Source: CAD feature listing. Evaluate the final solid. Frame: model axes, mm. Face numbers are marked on the shaded views. A direction names the side the tool comes from. Round coordinates to 2 decimals unless told otherwise and drop trailing zeros. Loops run counter-clockwise (first coordinate to the right, second up) from the corner with the lowest first, then second, coordinate; pieces in that order, holes last.
(1) Section D-D, the plane z = -1. Return the cut outline in (x, y) (3 decimals), plus the area to 3 significant figures.
(2) Set-up query: the marked faces 1, 2 and 3. Return all of +Z, -Z, +X, -X, +Y, -Y with unobstructed straight access to the full face (end or side cutting, diameter ignored); none if empty.
(3) Mould query, pull axis Y, two halves, no side actions, for the marked faces 4, 5, 6 and 7. Classes: pulls with the +Y half, pulls with the -Y half, needs draft (parallel to the pull), parting line crosses it, or undercut.
(4) Section A-A, the plane z = -6. Return the cut outline in (x, y) (3 decimals).
(5) Section C-C, the plane z = -23.83. Return the cut outline in (x, y) (3 decimals), plus the area to 3 significant figures.
(6) Section B-B, the plane x = 0. Return the cut outline in (y, z) (3 decimals), plus the area to 3 significant figures.
(7) First-contact query: pin 1 Ø8 at (x, y) = (-8, 2.5) entering from -Z; pin 2 Ø7.5 at (y, z) = (-7, -26) entering from -X; pin 3 Ø3.5 at (y, z) = (4, -11.5) entering from -X (3 decimals); pin 4 Ø6 at (x, z) = (-10.5, -26) entering from -Y. Flat tips, straight axial feed; report the tip coordinate or a pass-through.
(8) Material intervals for probe 1 along Y at (x, z) = (4.9, -23.83) (3 decimals); probe 2 along X at (y, z) = (7.5, -5) (3 decimals); probe 3 along X at (y, z) = (-2.5, -13.5) (3 decimals), sorted ascending.
```python
from build123d import *

# Parameters (mm, degrees)
SKETCH1_W           = 27
SKETCH1_H           = 27.25
BOSS_EXTRUDE1_DEPTH = 3.6
CHAMFER1_SIZE       = 2
BOSS_EXTRUDE2_DEPTH = 20.5
CUT_EXTRUDE1_START  = 3.6
SKETCH1_3_W         = 2.1
SKETCH1_3_H         = 8.7
SKETCH1_3_H_2       = 7
CUT_EXTRUDE1_DEPTH  = 22
SKETCH3_W           = 0.45
SKETCH3_H           = 9.6
SKETCH3_W_2         = 9.6
SKETCH3_H_2         = 0.45
BOSS_EXTRUDE3_DEPTH = 1.6
CHAMFER2_SIZE       = 1.5
SKETCH4_W           = 0.45
SKETCH4_H           = 4.85
BOSS_EXTRUDE4_DEPTH = 6.1
BOSS_EXTRUDE5_DEPTH = 2.4
SKETCH6_W           = 13.2
SKETCH6_H           = 0.85
BOSS_EXTRUDE6_DEPTH = 8.95
CHAMFER3_SIZE       = 1.2
CUT_EXTRUDE2_DEPTH  = 38.649057425
CUT_EXTRUDE3_REACH  = 35.476
BOSS_EXTRUDE7_DEPTH = 9.9
FILLET1_R           = 2


with BuildPart() as part:
    # Sketch1 → Boss-Extrude1 (new body)
    with BuildSketch(Plane.XY):
        Rectangle(SKETCH1_W, SKETCH1_H)
    extrude(amount=BOSS_EXTRUDE1_DEPTH)

    # Chamfer1
    chamfer1_edges = [part.edges().sort_by_distance(p)[0] for p in [
        (13.5, 0, 3.6),
        (0, -13.625, 3.6),
        (-13.5, 0, 3.6),
        (0, 13.625, 3.6),
    ]]
    chamfer(chamfer1_edges, length=CHAMFER1_SIZE)

    # Sketch2 → Boss-Extrude2 (add)
    with BuildSketch(Plane(origin=(0, 0, 0), x_dir=(-1, 0, 0), z_dir=(0, 0, -1))):
        Polygon((-8.625, 10.875), (8.625, 10.875), (8.625, -4.875), (4.325, -4.875), (4.325, -11.025), (-4.325, -11.025), (-4.325, -4.875), (-8.625, -4.875), align=None)
    extrude(amount=BOSS_EXTRUDE2_DEPTH)

    # Sketch1<3> → Cut-Extrude1 (cut)
    with BuildSketch(Plane.XY.offset(CUT_EXTRUDE1_START)):
        with Locations((-6.235, 4.725)):
            Rectangle(SKETCH1_3_W, SKETCH1_3_H)
        with Locations((6.235, 4.725)):
            Rectangle(SKETCH1_3_W, SKETCH1_3_H_2)
        with BuildLine():
            Line((2.65, -9.525), (2.65, -6.775))
            ThreePointArc((2.65, -6.775), (0, -4.125), (-2.65, -6.775))
            Line((-2.65, -6.775), (-2.65, -9.525))
            Line((-2.65, -9.525), (2.65, -9.525))
        make_face()
    extrude(amount=-CUT_EXTRUDE1_DEPTH, mode=Mode.SUBTRACT)

    # Sketch3 → Boss-Extrude3 (add)
    with BuildSketch(Plane(origin=(0, 0, -20.5), x_dir=(-1, 0, 0), z_dir=(0, 0, -1))):
        with Locations((-5.055, 4.325)):
            Rectangle(SKETCH3_W, SKETCH3_H)
        with Locations((5.055, 4.325)):
            Rectangle(SKETCH3_W, SKETCH3_H)
        with Locations((0, -4.3)):
            Rectangle(SKETCH3_W_2, SKETCH3_H_2)
    extrude(amount=BOSS_EXTRUDE3_DEPTH)

    # Chamfer2
    chamfer2_edges = [part.edges().sort_by_distance(p)[0] for p in [
        (-5.055, 9.125, -22.1),
        (5.055, 9.125, -22.1),
        (5.055, -0.475, -22.1),
        (-5.055, -0.475, -22.1),
    ]]
    chamfer(chamfer2_edges, length=CHAMFER2_SIZE)

    # Sketch4 → Boss-Extrude4 (add)
    with BuildSketch(Plane(origin=(0, 0, -22.1), x_dir=(-1, 0, 0), z_dir=(0, 0, -1))):
        with Locations((-5.055, 4.325)):
            Rectangle(SKETCH4_W, SKETCH4_H)
        with Locations((5.055, 4.325)):
            Rectangle(SKETCH4_W, SKETCH4_H)
    extrude(amount=BOSS_EXTRUDE4_DEPTH)

    # Sketch5 → Boss-Extrude5 (add, symmetric)
    with BuildSketch(Plane(origin=(0, 0, 0), x_dir=(0, 0, -1), z_dir=(1, 0, 0))):
        Polygon((22.1, -4.075), (29.65, -11.625), (29.331801948, -11.943198052), (21.913603897, -4.525), (22.1, -4.525), align=None)
    extrude(amount=BOSS_EXTRUDE5_DEPTH, both=True)

    # Sketch6 → Boss-Extrude6 (add)
    with BuildSketch(Plane(origin=(0, 0, -20.5), x_dir=(-1, 0, 0), z_dir=(0, 0, -1))):
        with Locations((0, -1.1)):
            Rectangle(SKETCH6_W, SKETCH6_H)
    extrude(amount=BOSS_EXTRUDE6_DEPTH)

    # Chamfer3
    chamfer3_edges = [part.edges().sort_by_distance(p)[0] for p in [
        (5.055, 6.75, -28.2),
        (5.055, 1.9, -28.2),
        (-5.055, 6.75, -28.2),
        (-5.055, 1.9, -28.2),
        (-2.4, -11.784099026, -29.490900974),
        (2.4, -11.784099026, -29.490900974),
    ]]
    chamfer(chamfer3_edges, length=CHAMFER3_SIZE)

    # Sketch7 → Cut-Extrude2 (cut, through all)
    with BuildSketch(Plane(origin=(5.28, 0, 0), x_dir=(0, 0, -1), z_dir=(1, 0, 0))):
        with BuildLine():
            Line((24.534285714, 5.592470565), (25.871428571, 4.849470579))
            ThreePointArc((25.871428571, 4.849470579), (26.18, 4.325), (25.871428571, 3.800529421))
            Line((25.871428571, 3.800529421), (24.534285714, 3.057529435))
            ThreePointArc((24.534285714, 3.057529435), (22.38, 4.325), (24.534285714, 5.592470565))
        make_face()
    extrude(amount=-CUT_EXTRUDE2_DEPTH, mode=Mode.SUBTRACT)

    # Sketch8 → Cut-Extrude3 (cut, up to next)
    with BuildSketch(Plane(origin=(0, 9.0125, -9.0125), x_dir=(1, 0, 0), z_dir=(0, 0.7071067811865465, -0.7071067811865487)), mode=Mode.PRIVATE) as cut_extrude3_sk1:
        with BuildLine():
            Line((-0.524470579, 26.857260965), (-1.267470565, 25.520118108))
            ThreePointArc((-1.267470565, 25.520118108), (0, 23.365832393), (1.267470565, 25.520118108))
            Line((1.267470565, 25.520118108), (0.524470579, 26.857260965))
            ThreePointArc((0.524470579, 26.857260965), (0, 27.165832393), (-0.524470579, 26.857260965))
        make_face()
    cut_extrude3_tool1 = extrude(cut_extrude3_sk1.sketch, amount=-CUT_EXTRUDE3_REACH, mode=Mode.PRIVATE) & part.part
    add(cut_extrude3_tool1.solids().sort_by_distance((0, -8.733008, -26.758008))[0], mode=Mode.SUBTRACT)

    # Sketch9 → Boss-Extrude7 (add)
    with BuildSketch(Plane.XZ.offset(4.875)):
        Polygon((-8.625, -18), (-10.525, -18), (-13.4644015, -4.29921357), (-14.075, -2.5), (-11.9, -0.36), (-11.9, -3.963582901), (-9.693125963, -14.25), (-8.625, -14.25), align=None)
    boss_extrude7 = extrude(amount=-BOSS_EXTRUDE7_DEPTH)

    # Mirror1: Boss-Extrude7 across plane
    add(boss_extrude7.mirror(Plane(origin=(0, 0, 0), x_dir=(0, 0, 1), z_dir=(1, 0, 0))))

    # Fillet1
    fillet1_edges = [part.edges().sort_by_distance(p)[0] for p in [
        (-10.525, 0.075, -18),
        (10.525, 0.075, -18),
    ]]
    fillet(fillet1_edges, radius=FILLET1_R)


solid = part.part
```
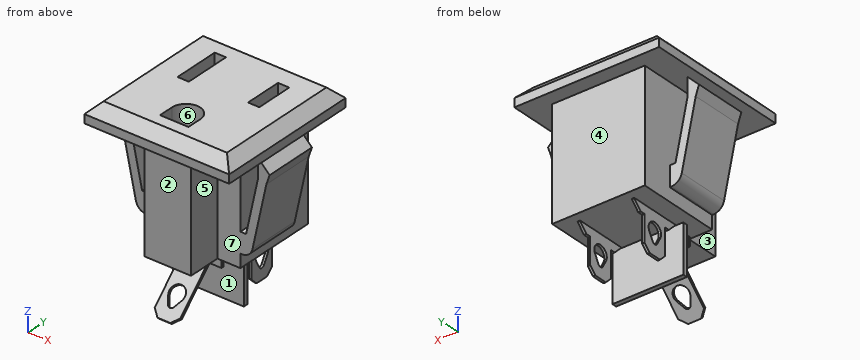
Output values:
1. outline: (-12.55, -4.875) - (-11.9, -4.875) - (-11.9, 5.025) - (-12.55, 5.025) - close; (-8.625, -4.875) - (-4.325, -4.875) - (-4.325, -11.025) - (4.325, -11.025) - (4.325, -4.875) - (8.625, -4.875) - (8.625, 10.875) - (-8.625, 10.875) - close; (11.9, -4.875) - (12.55, -4.875) - (12.55, 5.025) - (11.9, 5.025) - close; hole (-7.285, 0.375) - (-5.185, 0.375) - (-5.185, 9.075) - (-7.285, 9.075) - close; hole (-2.65, -9.525) - (2.65, -9.525) - (2.65, -6.775) arc R2.65 ccw to (-2.65, -6.775) - close; hole (5.185, 1.225) - (7.285, 1.225) - (7.285, 8.225) - (5.185, 8.225) - close
1. area: 279 mm2
2. face 1: -Z, +X, -X
2. face 2: +X, -X, -Y
2. face 3: -Z, -X, -Y
3. face 4: pulls with the +Y half
3. face 5: needs draft
3. face 6: undercut
3. face 7: pulls with the -Y half
4. outline: (-13.1, -4.875) - (-11.463, -4.875) - (-11.463, 5.025) - (-13.1, 5.025) - close; (-8.625, -4.875) - (-4.325, -4.875) - (-4.325, -11.025) - (4.325, -11.025) - (4.325, -4.875) - (8.625, -4.875) - (8.625, 10.875) - (-8.625, 10.875) - close; (11.463, -4.875) - (13.1, -4.875) - (13.1, 5.025) - (11.463, 5.025) - close; hole (-7.285, 0.375) - (-5.185, 0.375) - (-5.185, 9.075) - (-7.285, 9.075) - close; hole (-2.65, -9.525) - (2.65, -9.525) - (2.65, -6.775) arc R2.65 ccw to (-2.65, -6.775) - close; hole (5.185, 1.225) - (7.285, 1.225) - (7.285, 8.225) - (5.185, 8.225) - close
5. outline: (-6.6, -1.525) - (6.6, -1.525) - (6.6, -0.675) - (-6.6, -0.675) - close; (-5.28, 1.9) - (-4.83, 1.9) - (-4.83, 2.875) - (-5.28, 2.875) - close; (-5.28, 5.775) - (-4.83, 5.775) - (-4.83, 6.75) - (-5.28, 6.75) - close; (-2.4, -6.441) - (2.4, -6.441) - (2.4, -5.805) - (-2.4, -5.805) - close; (4.83, 1.9) - (5.28, 1.9) - (5.28, 2.875) - (4.83, 2.875) - close; (4.83, 5.775) - (5.28, 5.775) - (5.28, 6.75) - (4.83, 6.75) - close
5. area: 16.0 mm2
6. outline: (-13.625, 0) - (-11.025, 0) - (-11.025, -20.5) - (-4.525, -20.5) - (-4.525, -21.914) - (-7.828, -25.216) - (-7.51, -25.535) - (-4.075, -22.1) - (-4.075, -20.5) - (-1.525, -20.5) - (-1.525, -29.45) - (-0.675, -29.45) - (-0.675, -20.5) - (10.875, -20.5) - (10.875, 0) - (13.625, 0) - (13.625, 1.6) - (11.625, 3.6) - (-4.125, 3.6) - (-4.125, -18.4) - (-9.525, -18.4) - (-9.525, 3.6) - (-11.625, 3.6) - (-13.625, 1.6) - close; (-11.943, -29.332) - (-11.625, -29.65) - (-10.197, -28.222) - (-10.515, -27.903) - close
6. area: 436 mm2
7. pin 1: stops at z = -29.45
7. pin 2: stops at x = -2.4
7. pin 3: stops at x = -12.295
7. pin 4: passes through
8. probe 1: y = -1.525 to -0.675, 1.9 to 2.875, 5.775 to 6.75
8. probe 2: x = -8.625 to -7.285, -5.185 to 5.185, 7.285 to 8.625
8. probe 3: x = -11.49 to -9.854, -8.625 to 8.625, 9.854 to 11.49
